For this review, take the finished solid that the model builds, in its own axes (mm). Coordinates: 2 decimals unless noted, no trailing zeros. Write each loop counter-clockwise with the first axis right and the second up, starting at its lowest first coordinate (ties: lowest second). Pieces come first, ordered by that corner, then holes.
1) We need section C-C on y = 5. Write out the cut boundary in (x, z), then the cut area to 3 significant figures.
2) We need section B-B on z = 5. Write out the cut boundary in (x, y).
3) Insertion check: P1, Ø1.6, axis at y = -1.5, z = -12.5, coming from the -X side; P2, Ø1, axis at x = 32, y = -1.5, coming from the -Z side; P3, Ø1.6, axis at x = -12.5, y = -1.5, coming from the +Z side. Each pin has a flat end and moves straight along its axis. Give the tip position at first contact, or say it passes through.
4) To check wall thickness, follow line 1 along Z through (x, y) = (64.5, 6); line 2 along X through (y, z) = (6.25, -7). State the ranges of each line that lie inside material, in increasing order.
5) We need section A-A on x = -70. Write out the cut boundary in (y, z).
from build123d import *

# Parameters (mm, degrees)
F0_W         = 174.7
F0_H         = 108.2
F0_W_2       = 169.9
F0_H_2       = 103.4
F1_DEPTH     = 2
F0_W_3       = 167.5
F0_H_3       = 101
F2_DEPTH     = 7
F3_R         = 4
F4_R         = 5
F5_R         = 8
F6_T1_DEPTH  = 158.7
F6_T3_DEPTH  = 92.2
F6_T6_ANGLE  = 90
F6_T8_ANGLE  = 90
F6_T10_ANGLE = 90
F6_T12_ANGLE = 90


# Not quite as in the source:
# - a fillet or chamfer that OpenCascade refuses, or shapes differently, is made with other operations: its cross-section is extruded or revolved along the edge and cut away or added


with BuildPart() as f1:
    # F0 (on Front) → F1 (new body)
    with BuildSketch(Plane.XZ):
        Rectangle(F0_W, F0_H)
        Rectangle(F0_W_2, F0_H_2, mode=Mode.SUBTRACT)
    extrude(amount=F1_DEPTH)

    # F0 (on Front) → F2 (join)
    with BuildSketch(Plane.XZ):
        Rectangle(F0_W, F0_H)
        Rectangle(F0_W_2, F0_H_2, mode=Mode.SUBTRACT)
        Rectangle(F0_W_2, F0_H_2)
        Rectangle(F0_W_3, F0_H_3, mode=Mode.SUBTRACT)
    extrude(amount=-F2_DEPTH)

    # F3
    f3_edges = [f1.edges().sort_by_distance(p)[0] for p in [
        (83.75, 3.5, 50.5),
        (-83.75, 3.5, 50.5),
        (-83.75, 3.5, -50.5),
        (83.75, 3.5, -50.5),
    ]]
    fillet(f3_edges, radius=F3_R)

    # F4
    f4_edges = [f1.edges().sort_by_distance(p)[0] for p in [
        (84.95, -1, 51.7),
        (84.95, -1, -51.7),
        (-84.95, -1, -51.7),
        (-84.95, -1, 51.7),
    ]]
    fillet(f4_edges, radius=F4_R)

    # F5
    f5_edges = [f1.edges().sort_by_distance(p)[0] for p in [
        (87.35, 2.5, -54.1),
        (-87.35, 2.5, -54.1),
        (-87.35, 2.5, 54.1),
        (87.35, 2.5, 54.1),
    ]]
    fillet(f5_edges, radius=F5_R)

    # F6: fillet of radius 2.5 on 1 edges, made by hand

    # F6_s2 → F6_t1 (cut)
    with BuildSketch(Plane.YZ.offset(-79.35)):
        with BuildLine():
            ThreePointArc((-2, 51.6), (-1.267766953, 53.367766953), (0.5, 54.1))
            Line((0.5, 54.1), (-2, 54.1))
            Line((-2, 54.1), (-2, 51.6))
        make_face()
        with BuildLine():
            ThreePointArc((-2, -51.6), (-1.267766953, -53.367766953), (0.5, -54.1))
            Line((0.5, -54.1), (-2, -54.1))
            Line((-2, -54.1), (-2, -51.6))
        make_face()
    extrude(amount=F6_T1_DEPTH, mode=Mode.SUBTRACT)

    # F6_s4 → F6_t3 (cut)
    with BuildSketch(Plane.XY.offset(-46.1)):
        with BuildLine():
            ThreePointArc((-84.85, -2), (-86.617766953, -1.267766953), (-87.35, 0.5))
            Line((-87.35, 0.5), (-87.35, -2))
            Line((-87.35, -2), (-84.85, -2))
        make_face()
        with BuildLine():
            ThreePointArc((84.85, -2), (86.617766953, -1.267766953), (87.35, 0.5))
            Line((87.35, 0.5), (87.35, -2))
            Line((87.35, -2), (84.85, -2))
        make_face()
    extrude(amount=F6_T3_DEPTH, mode=Mode.SUBTRACT)

    # F6_s5 → F6_t6 (revolve, cut)
    with BuildSketch(Plane.YZ.offset(-79.35)):
        with BuildLine():
            ThreePointArc((-2, 51.6), (-1.267766953, 53.367766953), (0.5, 54.1))
            Line((0.5, 54.1), (-2, 54.1))
            Line((-2, 54.1), (-2, 51.6))
        make_face()
    revolve(axis=Axis((-79.35, -2, 46.1), (0, -1, 0)), revolution_arc=F6_T6_ANGLE, mode=Mode.SUBTRACT)

    # F6_s7 → F6_t8 (revolve, cut)
    with BuildSketch(Plane.XY.offset(-46.1)):
        with BuildLine():
            ThreePointArc((-84.85, -2), (-86.617766953, -1.267766953), (-87.35, 0.5))
            Line((-87.35, 0.5), (-87.35, -2))
            Line((-87.35, -2), (-84.85, -2))
        make_face()
    revolve(axis=Axis((-79.35, -2, -46.1), (0, -1, 0)), revolution_arc=F6_T8_ANGLE, mode=Mode.SUBTRACT)

    # F6_s9 → F6_t10 (revolve, cut)
    with BuildSketch(Plane.XY.offset(-46.1)):
        with BuildLine():
            ThreePointArc((84.85, -2), (86.617766953, -1.267766953), (87.35, 0.5))
            Line((87.35, 0.5), (87.35, -2))
            Line((87.35, -2), (84.85, -2))
        make_face()
    revolve(axis=Axis((79.35, -2, -46.1), (0, 1, 0)), revolution_arc=F6_T10_ANGLE, mode=Mode.SUBTRACT)

    # F6_s11 → F6_t12 (revolve, cut)
    with BuildSketch(Plane.XY.offset(46.1)):
        with BuildLine():
            ThreePointArc((84.85, -2), (86.617766953, -1.267766953), (87.35, 0.5))
            Line((87.35, 0.5), (87.35, -2))
            Line((87.35, -2), (84.85, -2))
        make_face()
    revolve(axis=Axis((79.35, -2, 46.1), (0, -1, 0)), revolution_arc=F6_T12_ANGLE, mode=Mode.SUBTRACT)


solid = f1.part
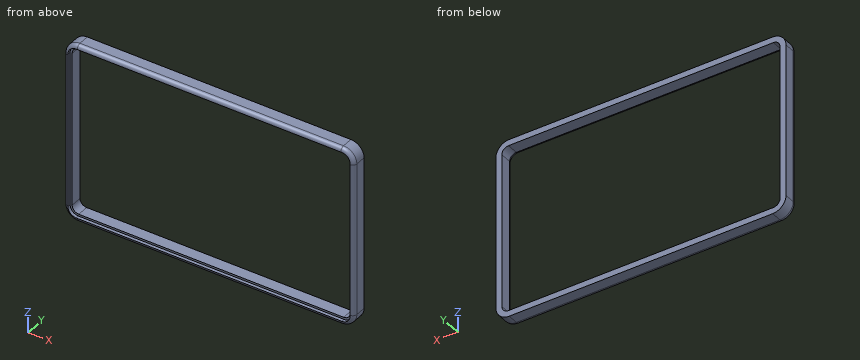
Result:
1. outline: (-87.35, -46.1) arc R8 ccw to (-79.35, -54.1) - (79.35, -54.1) arc R8 ccw to (87.35, -46.1) - (87.35, 46.1) arc R8 ccw to (79.35, 54.1) - (-79.35, 54.1) arc R8 ccw to (-87.35, 46.1) - close; hole (-83.75, -46.5) arc R4 ccw to (-79.75, -50.5) - (79.75, -50.5) arc R4 ccw to (83.75, -46.5) - (83.75, 46.5) arc R4 ccw to (79.75, 50.5) - (-79.75, 50.5) arc R4 ccw to (-83.75, 46.5) - close
1. area: 1,940 mm2
2. outline: (-87.35, 0.5) arc R2.5 ccw to (-84.95, -2) - (-84.95, 0) - (-83.75, 0) - (-83.75, 7) - (-87.35, 7) - close; (83.75, 0) - (84.95, 0) - (84.95, -2) arc R2.5 ccw to (87.35, 0.5) - (87.35, 7) - (83.75, 7) - close
3. P1: stops at x = -87.04
3. P2: stops at z = -53.6
3. P3: stops at z = 53.79
4. line 1: z = -54.1 to -50.5, 50.5 to 54.1
4. line 2: x = -87.35 to -83.75, 83.75 to 87.35
5. outline: (-2, -51.7) arc R2.5 ccw to (0.5, -54.1) - (7, -54.1) - (7, -50.5) - (0, -50.5) - (0, -51.7) - close; (-2, 51.7) - (0, 51.7) - (0, 50.5) - (7, 50.5) - (7, 54.1) - (0.5, 54.1) arc R2.5 ccw to start
